Autodesk Inventor part; units mm, degrees
ref_plane "YZ Plane" through (0, 0, 0) normal (1, 0, 0) x (0, 1, 0)
ref_plane "XZ Plane" through (0, 0, 0) normal (0, 1, 0) x (-1, 0, 0)
ref_plane "XY Plane" through (0, 0, 0) normal (0, 0, 1) x (1, 0, 0)
sketch "Sketch2" plane through (0, 0, 0) normal (0, 1, 0) x (-1, 0, 0)
  line L0 (-430.299, 15) -> (430.299, 15)
  line L1 (430.299, 15) -> (430.299, -15)
  line L2 (430.299, -15) -> (-430.299, -15)
  line L3 (-430.299, -15) -> (-430.299, 15)
  line L4 (-430.299, 15) -> (430.299, -15) construction
  line L5 (430.299, 15) -> (-430.299, -15) construction
  point P0 (0, 0)
  dimension "d12" = 860.598
  dimension "d13" = 30
extrude "Plate2" add sketch "Sketch2" along normal blind 1.5
sketch "Sketch3" plane through (-430.299, 0, 15) normal (0, 0, 1) x (1, 0, 0)
  line L0 (842.098, 0) -> (18.5, 0)
  line L1 (18.5, 0) -> (18.5, -18.5)
  line L2 (18.5, -18.5) -> (842.098, -18.5)
  line L3 (842.098, -18.5) -> (842.098, 0)
edge flange "Flange1" height 20 angle 90 thickness 1.5 bend radius 1.5 thickness toward (0, 0, 1) relief straight relief width 1.5 relief depth 0.75 edges at (0, 0, 15) wall of the first edge with corners at (411.799, 0, 15) (-411.799, 0, 15) (-411.799, -18.5, 15) (411.799, -18.5, 15)
bend "Bend2"
corner "Corner2"
sketch "Sketch4" plane through (430.299, 1.5, -13.5) normal (0, 0, -1) x (-1, 0, 0)
  line L0 (860.598, 0) -> (0, 0)
  line L1 (0, 0) -> (0, -10)
  line L2 (0, -10) -> (860.598, -10)
  line L3 (860.598, -10) -> (860.598, 0)
edge flange "Flange2" height 10 angle 90 thickness 1.5 bend radius 1.5 thickness toward (0, 0, -1) relief tear relief width 1.5 relief depth 0.75 edges at (0, 0, -15) wall of the first edge with corners at (-430.299, 1.5, -13.5) (430.299, 1.5, -13.5) (430.299, -8.5, -13.5) (-430.299, -8.5, -13.5)
bend "Bend3"
corner "Corner3"
sketch "Sketch5" plane through (411.799, -18.5, 15) normal (0, 0, -1) x (-1, 0, 0)
  circle A0 centre (391.799, 8.5) radius 2.067 construction
  circle A1 centre (431.799, 8.5) radius 2.067 construction
  circle A2 centre (391.799, 8.5) radius 2.75
  circle A3 centre (431.799, 8.5) radius 2.75
  point P0 (411.799, 18.5)
  dimension "d36" = 5.5
  dimension "d37" = 5.5
extrude "Extrusion1" cut sketch "Sketch5" against normal blind 1.5
chamfer "Chamfer1" distance 1.5 angle 45 2 edges at (22.75, -10, 16.5) (-17.25, -10, 16.5)
equation "\"d38\" = Thickness"
equation "\"d15\" = BendReliefWidth"
equation "\"d16\" = BendReliefDepth"
equation "\"d17\" = MinimumRemnant"
equation "\"d18\" = BendRadius"
equation "\"d22\" = BendRadius"
equation "\"d23\" = CornerReliefSize"
equation "\"d24\" = GapSize"
equation "\"d25\" = JacobiRadiusSize"
equation "\"d26\" = BendReliefWidth"
equation "\"d27\" = BendReliefDepth"
equation "\"d28\" = MinimumRemnant"
equation "\"d29\" = BendRadius"
equation "\"d32\" = BendRadius"
equation "\"d33\" = CornerReliefSize"
equation "\"d34\" = GapSize"
equation "\"d35\" = JacobiRadiusSize"
equation "\"BendRadius\" = Thickness"
equation "\"BendReliefWidth\" = Thickness"
equation "\"BendReliefDepth\" = 0.5 * Thickness"
equation "\"CornerReliefSize\" = 4 * Thickness"
equation "\"MinimumRemnant\" = 2 * Thickness"
equation "\"TransitionRadius\" = BendRadius"
equation "\"JacobiRadiusSize\" = BendRadius"
equation "\"GapSize\" = Thickness"
equation "\"d14\" = BendRadius"
properties part number "Batente Sup." material "Stainless Steel"
Source: CAD feature listing. Evaluate the final solid. Frame: model axes, mm. Give positions to 0.01 mm unless a question says otherwise; leave off trailing zeros. Order: outer loops, then holes, each group sorted by start corner. A loop starts at its lowest first (then second) coordinate and runs counter-clockwise, first axis right, second up.
(1) Material intervals for line 1 along Z through (x, y) = (-368.5, -4.25); line 2 along X through (y, z) = (-10, 15.05); line 3 along Z through (x, y) = (-376, -14), sorted ascending.
(2) Section query A-A (x = -67). Return the cut outline in (y, z), plus the area to 3 significant figures.
(3) Pull-direction query (Z, two-part tool) for faces 1 (the face through (-6, -10, 16.5)), 2 (the face through (6, 0, 2)), 3 (the face through (6, 1.5, 2)); classes: +Z half, -Z half, draft (parallel to the pull), parting line (faces both ways), or undercut.
(4) Contact query for flat-ended pins moving along their axis: P1, Ø2, axis at y = -2.5, z = 4.5, coming from the +X side; P2, Ø5, axis at x = -255, y = -9, coming from the -Z side; P3, Ø4.5, axis at x = 20, y = -10, coming from the +Z side; P4, Ø0.8, axis at x = -412.5, y = 0.5, coming from the +Z side. Output: stop coordinate, or through.
Outcome:
1. line 1: z = -15 to -13.5, 15 to 16.5
1. line 2: x = -411.8 to -22.8, -17.2 to 17.2, 22.8 to 411.8
1. line 3: z = 15 to 16.5
2. outline: (-18.5, 15) - (-1.5, 15) arc R1.5 cw to (0, 13.5) - (0, -12) arc R1.5 cw to (-1.5, -13.5) - (-8.5, -13.5) - (-8.5, -15) - (-1.5, -15) arc R3 ccw to (1.5, -12) - (1.5, 13.5) arc R3 ccw to (-1.5, 16.5) - (-18.5, 16.5) - close
2. area: 84.9 mm2
3. face 1: +Z half
3. face 2: undercut
3. face 3: draft
4. P1: passes through
4. P2: stops at z = -15
4. P3: stops at z = -13.5
4. P4: stops at z = 12.75
